The figure shows three views and two pictorial views of one solid part (mm, origin at its lowest corner). Answer the questions. A direction names the side the tool comes from. Coordinates: 2 decimals unless noted, no trailing zeros. Loops run counter-clockwise (first coordinate to the right, second up) from the corner with the lowest first, then second, coordinate; pieces in that order, holes last. Notation, with made-up numbers: (76.25, 83.5) - (95.25, 83.5) arc R36 cw to (95.25, 119.5) - close; hole circle Ø4 at (63.5, -27.5). An arc over 180 degrees is marked (long way). Return JSON: item names as keys, results as strings. Group by question number.
1. Which of the six approach directions +Z, -Z, +X, -X, +Y, -Y give full straight-line access (tool end or side, diameter ignored) to the marked faces 1 and 2?
2. Section D-D (z = 44) is taken. Write down the section's boundary in (x, y), and give its area (3 significant figures).
3. Section C-C (x = 25) is taken. State how many separate pieces and enclosed holes the cut face has, and give its area (3 significant figures).
4. Find the intervals of material crossed by line 1 along Z through (x, y) = (28, 11); line 2 along Y through (x, z) = (25, 71.6); line 3 along Y through (x, z) = (5, 72), in increasing order.
5. Section A-A (x = 45) is taken. Write down the section's boundary in (y, z), and give its area (3 significant figures).
6. The mould has two halves that part along X. Classify the marked faces 3, 4 and 5: pulls with the +X half, pulls with the -X half, needs draft (parallel to the pull), parting line crosses it, or undercut.
7. Each of these flat-tipped pins is pushed along its axis until it touches: P1, Ø4, axis at x = 35.5, z = 60.5, coming from the -Y side; P2, Ø10, axis at y = 39, z = 10.5, coming from the +X side; P3, Ø6, axis at y = 38, z = 34, coming from the -X side; P4, Ø15, axis at x = 26, y = 26, coming from the +Z side. Where does it stop, or does it pass through?
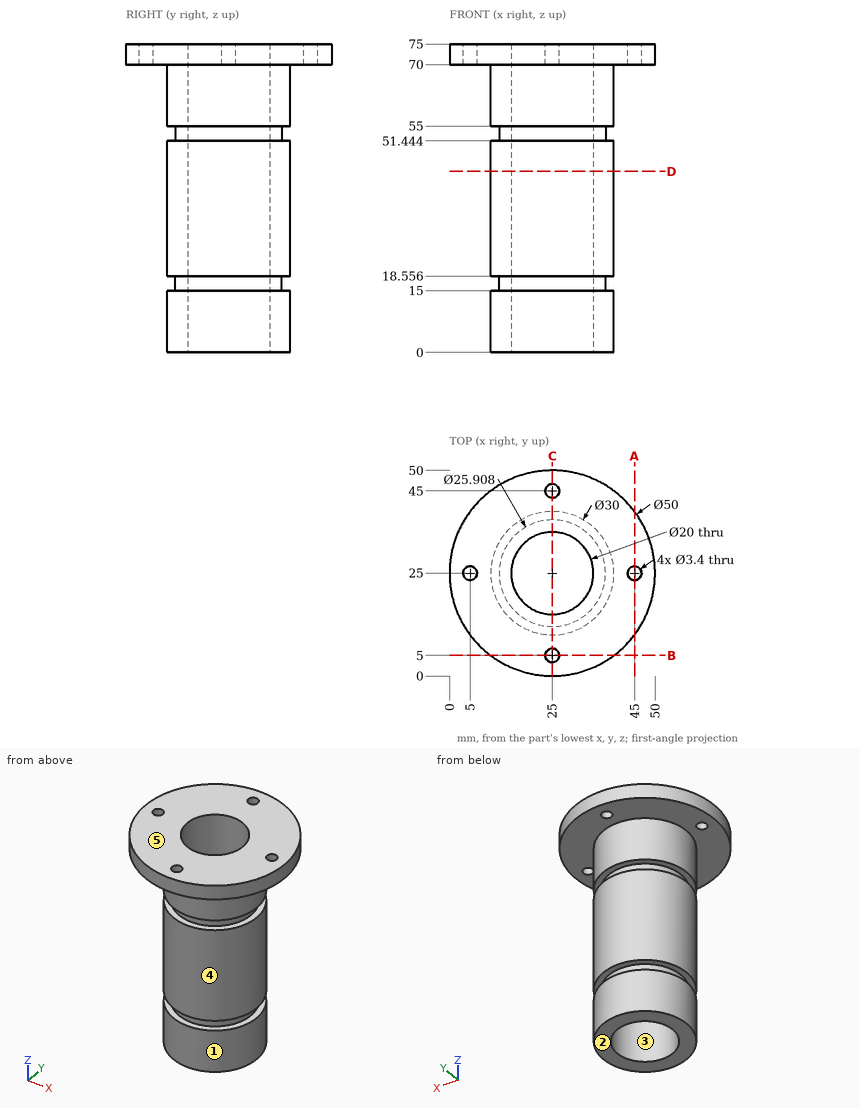
The answers:
{
 "1": {"face 1": "-Z", "face 2": "-Z, +X, -X, +Y, -Y"},
 "2": {"outline": "circle Ø30 at (25, 25); hole circle Ø20 at (25, 25)", "area": "393 mm2"},
 "3": {"separate pieces": "4", "enclosed holes": "0", "area": "787 mm2"},
 "4": {"line 1": "z = 0 to 15, 18.56 to 51.44, 55 to 75", "line 2": "y = 0 to 3.3, 6.7 to 15, 35 to 43.3, 46.7 to 50", "line 3": "y = 10 to 23.3, 26.7 to 40"},
 "5": {"outline": "(10, 70) - (23.3, 70) - (23.3, 75) - (10, 75) - close; (26.7, 70) - (40, 70) - (40, 75) - (26.7, 75) - close", "area": "133 mm2"},
 "6": {"face 3": "undercut", "face 4": "parting line crosses it", "face 5": "needs draft"},
 "7": {"P1": "stops at y = 12.64", "P2": "stops at x = 37", "P3": "stops at x = 13.82", "P4": "passes through"}
}
